Autodesk Inventor part; units mm, degrees
ref_plane "Work Plane1" through (5.2, 0, 0) normal (1, 0, 0) x (0, 0, -1)
ref_plane "YZ Plane" through (0, 0, 0) normal (1, 0, 0) x (0, 1, 0)
ref_plane "XZ Plane" through (0, 0, 0) normal (0, 1, 0) x (-1, 0, 0)
sketch "Sketch1" plane through (0, 0, 0) normal (0, 0, 1) x (1, 0, 0)
  line L0 (0, 0) -> (10.4, 0)
  line L1 (10.4, 0) -> (10.4, 10.4)
  line L2 (10.4, 10.4) -> (0, 10.4)
  line L3 (0, 10.4) -> (0, 0)
  line L4 (-2, 12.4) -> (12.4, 12.4)
  line L5 (12.4, 12.4) -> (12.4, -2)
  line L6 (12.4, -2) -> (-2, -2)
  line L7 (-2, -2) -> (-2, 12.4)
  dimension "d0" = 10.4
  dimension "d1" = 10.4
  dimension "d2" = 2
extrude "Extrusion1" add sketch "Sketch1" along normal blind 1
sketch "Sketch2" plane through (12.4, -2, 0) normal (1, 0, 0) x (0, 0, -1)
  line L0 (0, 14.4) -> (-1, 14.4)
  line L1 (-1, 14.4) -> (-4.5, 4.5)
  line L2 (-4.5, 4.5) -> (-4.5, 0)
  line L3 (0, 0) -> (-1, 0)
  line L4 (-4.5, 0) -> (-1, 0)
  line L5 (-1, 0) -> (-1, 14.4)
  line L6 (-1, 14.4) -> (-4.5, 14.4)
  line L7 (-4.5, 14.4) -> (-4.5, 4.5)
  point P0 (0, 2)
  dimension "d5" = 4.5
  dimension "d6" = 4.5
extrude "Extrusion3" add sketch "Sketch2" against normal up to surface (2 mm away) contours L5 L4 L2 L1
ref_plane "Work Plane1" through (5.2, 0, 0) normal (1, 0, 0) x (0, 0, -1)
mirror "Mirror1" about plane through (5.2, 0, 0) normal (1, 0, 0) of "Extrusion3"
sketch "Sketch5" plane through (-2, -2, 0) normal (0, -1, 0) x (1, 0, 0)
  line L0 (14.4, 0) -> (0, 0)
  line L1 (14.4, 0) -> (14.4, 4.5)
  line L2 (0, 0) -> (14.4, 0)
  line L3 (14.4, 0) -> (14.4, 4.5)
  line L4 (14.4, 4.5) -> (0, 4.5)
  line L5 (0, 4.5) -> (0, 0)
  point P0 (2, 0)
extrude "Extrusion4" add sketch "Sketch5" against normal blind 2
sketch "Sketch6" plane through (0, 0, 0) normal (0, 0, -1) x (-1, 0, 0)
  line L0 (-7.2, 3) -> (-3.2, 3)
  line L1 (-3.2, 3) -> (-3.2, 0)
  line L2 (-3.2, 0) -> (-7.2, 0)
  line L3 (-7.2, 0) -> (-7.2, 3)
  line L4 (-12.4, -2) -> (2, -2)
  line L5 (-7.2, 3) -> (-12.4, 3)
  line L6 (-3.2, 3) -> (2, 3)
  line L7 (-10.4, -2) -> (0, -2)
  line L8 (-12.4, 3) -> (-12.4, -2)
  line L9 (2, 3) -> (2, -2)
  point P0 (0, 0)
  point P1 (-5.2, 3)
  point P2 (-5.2, -2)
  dimension "d15" = 4
  dimension "d16" = 3
  dimension "d17" = 2
extrude "Extrusion5" add sketch "Sketch6" along normal blind 8 contours L0 L1 L2 L3
extrude "Extrusion6" add sketch "Sketch6" along normal blind 2 contours L3 L2 L1 L6 L9 L4 L8 L5
sketch "Sketch4" plane through (-2, -2, 0) normal (0, -1, 0) x (1, 0, 0)
  line L0 (14.4, 1) -> (0, 1)
  line L1 (0, 1) -> (14.4, 1)
  line L2 (0, 1) -> (0, 4.5)
  line L3 (0, 4.5) -> (2, 4.5)
  line L4 (2, 4.5) -> (2, 3)
  line L5 (2, 3) -> (12.4, 3)
  line L6 (12.4, 3) -> (12.4, 4.5)
  line L7 (12.4, 4.5) -> (14.4, 4.5)
  line L8 (14.4, 4.5) -> (14.4, 1)
  point P0 (2, 0)
  point P1 (12.4, 1)
  point P2 (2, 1)
  dimension "d8" = 2
properties part number "Encoder Mount" material "ABS Plastic"
Input: part model. Units: mm. Frame: model coordinates. A direction names the side the tool comes from. Coordinates: 2 decimals unless noted, no trailing zeros. Loops run counter-clockwise (first coordinate to the right, second up) from the corner with the lowest first, then second, coordinate; pieces in that order, holes last. Notation, with made-up numbers: M 73,37.5 L 100,37.5 A17 ccw 100,66.5 Z; hole C 28.5,-5.75 d2. An arc over 180 degrees is marked long. Use a Markdown table: item, result. Add a question column.
1) Section B-B, the plane y = 5.75. Return the cut outline in (x, z).
2) Section C-C, the plane x = 5.75. Return the cut outline in (y, z), plus the area to 3 significant figures.
3) Line query: L1, parallel to X at y = 0.75, z = -3; L2, parallel to Z at x = 6.5, y = 2.25; L3, parallel to Y at x = 4.5, z = 3.5. Output: solid intervals per line, ascending. Write a range as from..to.
4) Set-up query: faces 1 (the flat face through (5, 0, -5)), 2 (the flat face through (5, 11, 1)), 3 (the flat face through (10.4, 5, 2)), 4 (the flat face through (5.3, 10.4, 0.5)). Return all of +Z, -Z, +X, -X, +Y, -Y with unobstructed straight access to the full face (end or side cutting, diameter ignored); none if empty.
5) Section D-D, the plane y = 1.5. Return the cut outline in (x, z), plus the area to 3 significant figures.
6) Pin query (flat end, axial travel): P1, Ø1.5, axis at x = 7.5, y = 1, coming from the +Z side; P2, Ø0.9, axis at y = 2, z = -6, coming from the +X side; P3, Ø6, axis at x = 0.5, y = 10.5, coming from the +Z side; P4, Ø2, axis at x = 7.5, y = 5.5, coming from the +Z side. Return the tip coordinate at first contact, or that it passes through.
7) Draft query along X for faces 5 (the flat face through (7.2, 1, -5)), 6 (the flat face through (5, -1, 4.5)), 7 (the flat face through (5, 2, 0)). Return one class per face: +X half, -X half, draft (parallel to the pull), parting line (faces both ways), or undercut.
8) Section A-A, the plane x = 0.75. Return the cut outline in (y, z).
Answer below:
| question | item | result |
|---|---|---|
| 1 | outline | M -2,0 L 0,0 L 0,3.35 L -2,3.35 Z; M 10.4,0 L 12.4,0 L 12.4,3.35 L 10.4,3.35 Z |
| 2 | outline | M -2,-2 L 0,-2 L 0,-8 L 3,-8 L 3,0 L 0,0 L 0,4.5 L -2,4.5 Z; M 10.4,0 L 12.4,0 L 12.4,1 L 10.4,1 Z |
| 2 | area | 39.0 mm2 |
| 3 | L1 | 3.2..7.2 |
| 3 | L2 | -8..0 |
| 3 | L3 | -2..0 |
| 4 | face 1 | -Z, +X, -X, -Y |
| 4 | face 2 | +Z, +Y |
| 4 | face 3 | +Z |
| 4 | face 4 | +Z, -Z |
| 5 | outline | M -2,-2 L 3.2,-2 L 3.2,-8 L 7.2,-8 L 7.2,-2 L 12.4,-2 L 12.4,4.5 L 10.4,4.5 L 10.4,0 L 0,0 L 0,4.5 L -2,4.5 Z |
| 5 | area | 70.8 mm2 |
| 6 | P1 | z = 0 |
| 6 | P2 | x = 7.2 |
| 6 | P3 | z = 2.72 |
| 6 | P4 | through |
| 7 | face 5 | +X half |
| 7 | face 6 | draft |
| 7 | face 7 | undercut |
| 8 | outline | M -2,-2 L 3,-2 L 3,0 L 0,0 L 0,4.5 L -2,4.5 Z; M 10.4,0 L 12.4,0 L 12.4,1 L 10.4,1 Z |
